The listing builds one solid part. Answer for the finished solid, in the listing's coordinates (mm). Coordinates: 2 decimals unless noted, no trailing zeros. Order: outer loops, then holes, each group sorted by start corner. A loop starts at its lowest first (then second) coordinate and runs counter-clockwise, first axis right, second up. Notation, with made-up numbers: (30.5, 25.5) -> (60.5, 25.5) arc R15 cw to (60.5, 34.5) -> close; hole circle Ø10 at (53.25, -16.75). An arc over 180 degrees is marked (long way). Answer in a Markdown table with one row per item.
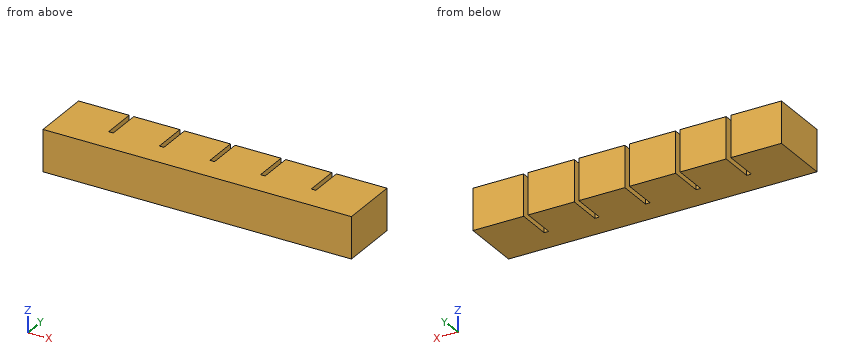
```python
from build123d import *

# Parameters (mm, degrees)
SKETCH1_W           = 20
SKETCH1_H           = 20
BOSS_EXTRUDE1_DEPTH = 18
SKETCH2_W           = 8
SKETCH2_H           = 6
CUT_EXTRUDE1_DEPTH  = 14
SKETCH3_W           = 18
SKETCH3_H           = 5
BOSS_EXTRUDE2_DEPTH = 2
LPATTERN1_COUNT     = 6
LPATTERN1_PITCH     = 22
SKETCH4_W           = 18
SKETCH4_H           = 15
BOSS_EXTRUDE3_DEPTH = 2
SKETCH5_W           = 18
SKETCH5_H           = 20
BOSS_EXTRUDE4_DEPTH = 2
SKETCH6_W           = 118
SKETCH6_H           = 2
CUT_EXTRUDE2_DEPTH  = 2
SKETCH7_W           = 134
SKETCH7_H           = 18
BOSS_EXTRUDE5_DEPTH = 6


with BuildPart() as part:
    # Sketch1 → Boss-Extrude1 (new body)
    with BuildSketch(Plane.XY):
        with Locations((10, 10)):
            Rectangle(SKETCH1_W, SKETCH1_H)
    extrude(amount=BOSS_EXTRUDE1_DEPTH)

    # Sketch2 → Cut-Extrude1 (cut)
    with BuildSketch(Plane(origin=(0, 0, 0), x_dir=(-1, 0, 0), z_dir=(0, -1, 0))):
        with Locations((-10, -9)):
            Rectangle(SKETCH2_W, SKETCH2_H)
    extrude(amount=-CUT_EXTRUDE1_DEPTH, mode=Mode.SUBTRACT)

    # Sketch3 → Boss-Extrude2 (add)
    with BuildSketch(Plane(origin=(20, 0, 0), x_dir=(0, 0, -1), z_dir=(1, 0, 0))):
        with Locations((-9, 2.5)):
            Rectangle(SKETCH3_W, SKETCH3_H)
    extrude(amount=BOSS_EXTRUDE2_DEPTH)


with BuildPart() as lpattern1_1:
    # LPattern1: pattern copy
    add(part.part.moved(Location(Vector(1, 0, 0) * (1 * LPATTERN1_PITCH))))


with BuildPart() as lpattern1_2:
    # LPattern1: pattern copy
    add(part.part.moved(Location(Vector(1, 0, 0) * (2 * LPATTERN1_PITCH))))


with BuildPart() as lpattern1_3:
    # LPattern1: pattern copy
    add(part.part.moved(Location(Vector(1, 0, 0) * (3 * LPATTERN1_PITCH))))


with BuildPart() as lpattern1_4:
    # LPattern1: pattern copy
    add(part.part.moved(Location(Vector(1, 0, 0) * (4 * LPATTERN1_PITCH))))


with BuildPart() as lpattern1_5:
    # LPattern1: pattern copy
    add(part.part.moved(Location(Vector(1, 0, 0) * (5 * LPATTERN1_PITCH))))

    # Sketch4 → Boss-Extrude3 (add)
    with BuildSketch(Plane(origin=(130, 0, 0), x_dir=(0, 0, -1), z_dir=(1, 0, 0))):
        with Locations((-9, 12.5)):
            Rectangle(SKETCH4_W, SKETCH4_H)
    extrude(amount=BOSS_EXTRUDE3_DEPTH)


with BuildPart() as part_1:
    add(part.part)

    # Sketch5 → Boss-Extrude4 (add)
    with BuildSketch(Plane.ZY):
        with Locations((9, 10)):
            Rectangle(SKETCH5_W, SKETCH5_H)
    extrude(amount=BOSS_EXTRUDE4_DEPTH)


with BuildPart() as lpattern1_4_1:
    add(lpattern1_4.part)

    # Combine1: union LPattern1_5, part, LPattern1_1, LPattern1_2, LPattern1_3
    add(lpattern1_5.part)
    add(part_1.part)
    add(lpattern1_1.part)
    add(lpattern1_2.part)
    add(lpattern1_3.part)

    # Sketch6 → Cut-Extrude2 (cut)
    with BuildSketch(Plane(origin=(0, 0, 0), x_dir=(-1, 0, 0), z_dir=(0, -1, 0))):
        with Locations((-65, -9)):
            Rectangle(SKETCH6_W, SKETCH6_H)
    extrude(amount=-CUT_EXTRUDE2_DEPTH, mode=Mode.SUBTRACT)

    # Sketch7 → Boss-Extrude5 (add)
    with BuildSketch(Plane(origin=(0, 0, 0), x_dir=(-1, 0, 0), z_dir=(0, -1, 0))):
        with Locations((-65, -9)):
            Rectangle(SKETCH7_W, SKETCH7_H)
    extrude(amount=BOSS_EXTRUDE5_DEPTH)


solid = lpattern1_4_1.part
```
(1) A cutting plane is placed at B-B, the plane x = 51.5. Determine the outline of the cut face in (y, z).
Check values:
| item | result |
|---|---|
| outline | (-6, 0) -> (20, 0) -> (20, 18) -> (-6, 18) -> close; hole (0, 6) -> (14, 6) -> (14, 12) -> (0, 12) -> close |
(2) A flat-ended cylindrical pin translates along its axis: pin 1 (1 mm diameter, centred on x = 65, z = 6.5, fed in from +Y). Find the tip coordinate at first contact, or state that the pin passes through.
Check values:
| item | result |
|---|---|
| pin 1 | y = 5 |
(3) A cutting plane is placed at D-D, the plane y = 8.75. Count the separate pieces of the cut face and the enclosed holes in it, then the cut area to 3 significant figures.
Check values:
| item | result |
|---|---|
| separate pieces | 6 |
| enclosed holes | 6 |
| area | 1,940 mm² |
(4) A cutting plane is placed at A-A, the plane y = 16. Determine the outline of the cut face in (x, z).
Check values:
| item | result |
|---|---|
| outline | (-2, 0) -> (20, 0) -> (20, 18) -> (-2, 18) -> close; (22, 0) -> (42, 0) -> (42, 18) -> (22, 18) -> close; (44, 0) -> (64, 0) -> (64, 18) -> (44, 18) -> close; (66, 0) -> (86, 0) -> (86, 18) -> (66, 18) -> close; (88, 0) -> (108, 0) -> (108, 18) -> (88, 18) -> close; (110, 0) -> (132, 0) -> (132, 18) -> (110, 18) -> close |
(5) A cutting plane is placed at C-C, the plane y = 3.75. Determine the outline of the cut face in (x, z), then the cut area to 3 significant figures.
Check values:
| item | result |
|---|---|
| outline | (-2, 0) -> (132, 0) -> (132, 18) -> (-2, 18) -> close; hole (6, 6) -> (14, 6) -> (14, 12) -> (6, 12) -> close; hole (28, 6) -> (36, 6) -> (36, 12) -> (28, 12) -> close; hole (50, 6) -> (58, 6) -> (58, 12) -> (50, 12) -> close; hole (72, 6) -> (80, 6) -> (80, 12) -> (72, 12) -> close; hole (94, 6) -> (102, 6) -> (102, 12) -> (94, 12) -> close; hole (116, 6) -> (124, 6) -> (124, 12) -> (116, 12) -> close |
| area | 2,120 mm² |
(6) Find the intervals of material crossed by line 1 along X through (y, z) = (14.25, 3.75); line 2 along Y through (x, z) = (96, 6.5); line 3 along Z through (x, y) = (123.5, 5.5), in increasing order. Write a range as from..to.
Check values:
| item | result |
|---|---|
| line 1 | -2..20, 22..42, 44..64, 66..86, 88..108, 110..132 |
| line 2 | -6..0, 14..20 |
| line 3 | 0..6, 12..18 |
